Can you work these out from the model? Positions are in its coordinate system, mm. Face numbers are marked on the shaded views. Round coordinates to 2 decimals unless told otherwise and drop trailing zeros. Loops run counter-clockwise (first coordinate to the right, second up) from the corner with the lowest first, then second, coordinate; pieces in that order, holes last.
from build123d import *

# Parameters (mm, degrees)
EXTRUDE_1_DEPTH      = 19
M8X1_251_D           = 6.8
M8X1_251_DEPTH       = 28.25
M8X1_251_CSINK_D     = 8.5
M8X1_251_CSINK_ANGLE = 90
M8X1_251_TIP         = 2.042926105


with BuildPart() as part:
    # Эскиз1 → Бобышка-Вытянуть1 (new body)
    with BuildSketch(Plane(origin=(0, 0, 0), x_dir=(0, 0, -1), z_dir=(1, 0, 0))):
        with BuildLine():
            Line((-6, 9.4), (-25.1, 9.4))
            Line((-25.1, 9.4), (-25.1, 50.6))
            Line((-25.1, 50.6), (-6, 50.6))
            ThreePointArc((-6, 50.6), (-1.757359313, 48.842640687), (0, 44.6))
            Line((0, 44.6), (0, 15.4))
            ThreePointArc((0, 15.4), (-1.757359313, 11.157359313), (-6, 9.4))
        make_face()
    extrude(amount=-EXTRUDE_1_DEPTH)

    # Отверстие обработанное метчиком M8x1.251
    with Locations(Plane(origin=(0, 0, 0), x_dir=(-1, 0, 0), z_dir=(0, 0, -1))):
        with Locations((9.5, 30)):
            CounterSinkHole(M8X1_251_D / 2, M8X1_251_CSINK_D / 2, depth=M8X1_251_DEPTH, counter_sink_angle=M8X1_251_CSINK_ANGLE)
            with Locations((0, 0, -(M8X1_251_DEPTH + M8X1_251_TIP / 2))):  # 118° drill point
                Cone(0, M8X1_251_D / 2, M8X1_251_TIP, mode=Mode.SUBTRACT)


solid = part.part
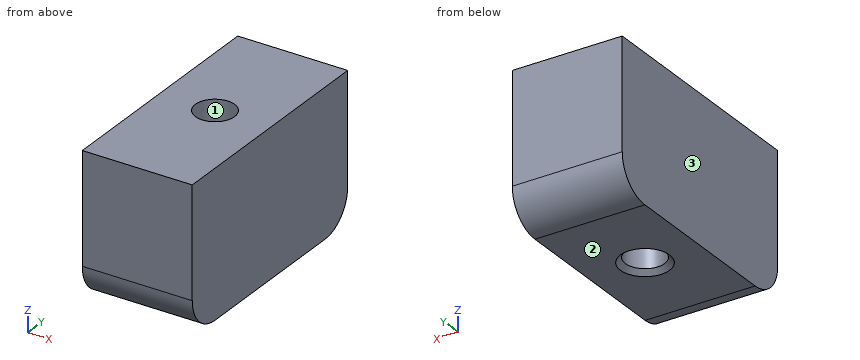
(1) Will this pin go through, and if not, where does the flat tip stop? P1, Ø5.5, axis at x = -9.5, y = 30, coming from the -Z side.
Worked answers:
P1: passes through
(2) If we mould it in two halves opening along X, with no side actions, what happens to the marked faces 1, 2 and 3? For each: released by +X, released by -X, zero draft, split by the parting line, or undercut.
Worked answers:
face 1: undercut
face 2: zero draft
face 3: released by -X
(3) If we section it at B-B, the plane y = 30: List the corners of the cut face in (x, z) for me, then the cut area to 3 significant figures.
Worked answers:
outline: (-19, 0) - (-13.75, 0) - (-12.9, 0.85) - (-12.9, 25.1) - (-19, 25.1) - close; (-6.1, 0.85) - (-5.25, 0) - (0, 0) - (0, 25.1) - (-6.1, 25.1) - close
area: 305 mm2
(4) If we section it at C-C, the plane z = 11.5: List the corners of the cut face in (x, y) for me.
Worked answers:
outline: (-19, 9.4) - (0, 9.4) - (0, 50.6) - (-19, 50.6) - close; hole circle Ø6.8 at (-9.5, 30)
(5) If I drill on line 1 (X direction, y = 30, z = 9.5); line 2 (Y direction, x = -9.5, z = 15.25); line 3 (Y direction, x = -8, z = 22.75), over which ranges is the centre line in solid material (lowest first)?
Worked answers:
line 1: x = -19 to -12.9, -6.1 to 0
line 2: y = 9.4 to 26.6, 33.4 to 50.6
line 3: y = 9.4 to 26.95, 33.05 to 50.6
(6) If we section it at A-A, the plane x = -9.5: List the corners of the cut face in (y, z) for me.
Worked answers:
outline: (9.4, 6) arc R6 ccw to (15.4, 0) - (25.75, 0) - (26.6, 0.85) - (26.6, 25.1) - (9.4, 25.1) - close; (33.4, 0.85) - (34.25, 0) - (44.6, 0) arc R6 ccw to (50.6, 6) - (50.6, 25.1) - (33.4, 25.1) - close
